The model under review builds one solid part; all positions refer to its coordinate system, in mm. Coordinates: 2 decimals unless noted, no trailing zeros. Loops run counter-clockwise (first coordinate to the right, second up) from the corner with the lowest first, then second, coordinate; pieces in that order, holes last. Notation, with made-up numbers: M -23.75,-17 L 35.25,-17 A28 ccw 35.25,8 Z; hole C 43,67 d2. An arc over 180 degrees is marked long. Return JSON: item names as keys, results as strings.
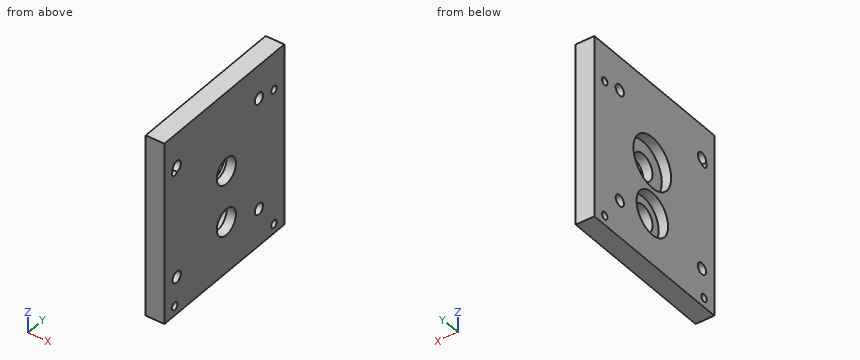
```python
from build123d import *

# Parameters (mm, degrees)
SKETCH1_W           = 20
SKETCH1_H           = 196
BOSS_EXTRUDE1_DEPTH = 175
SKETCH2_R           = 27.5
SKETCH2_R_2         = 23
CUT_EXTRUDE1_DEPTH  = 10
SKETCH3_R           = 14
CUT_EXTRUDE2_DEPTH  = 11
SKETCH4_R           = 4
CUT_EXTRUDE3_DEPTH  = 21
SKETCH5_R           = 6
CUT_EXTRUDE4_DEPTH  = 21


with BuildPart() as part:
    # Sketch1 → Boss-Extrude1 (new body)
    with BuildSketch(Plane(origin=(114, 0, 0), x_dir=(1, 0, 0), z_dir=(0, 1, 0))):
        with Locations((-114, 0)):
            Rectangle(SKETCH1_W, SKETCH1_H)
    extrude(amount=BOSS_EXTRUDE1_DEPTH)

    # Sketch2 → Cut-Extrude1 (cut)
    with BuildSketch(Plane.ZY.offset(10)):
        with Locations((12.5, 90.5)):
            Circle(SKETCH2_R)
        with Locations((-43, 90.5)):
            Circle(SKETCH2_R_2)
    extrude(amount=-CUT_EXTRUDE1_DEPTH, mode=Mode.SUBTRACT)

    # Sketch3 → Cut-Extrude2 (cut, through all)
    with BuildSketch(Plane.ZY):
        with Locations((12.5, 90.5)):
            Circle(SKETCH3_R)
        with Locations((-43, 90.5)):
            Circle(SKETCH3_R)
    extrude(amount=-CUT_EXTRUDE2_DEPTH, mode=Mode.SUBTRACT)

    # Sketch4 → Cut-Extrude3 (cut, through all)
    with BuildSketch(Plane.ZY.offset(10)):
        with Locations((58, 15)):
            Circle(SKETCH4_R)
        with Locations((-88, 15)):
            Circle(SKETCH4_R)
        with Locations((-88, 160)):
            Circle(SKETCH4_R)
        with Locations((58, 160)):
            Circle(SKETCH4_R)
    extrude(amount=-CUT_EXTRUDE3_DEPTH, mode=Mode.SUBTRACT)

    # Sketch5 → Cut-Extrude4 (cut, through all)
    with BuildSketch(Plane.ZY.offset(10)):
        with Locations((62, 138)):
            Circle(SKETCH5_R)
        with Locations((62, 18)):
            Circle(SKETCH5_R)
        with Locations((-58, 138)):
            Circle(SKETCH5_R)
        with Locations((-58, 18)):
            Circle(SKETCH5_R)
    extrude(amount=-CUT_EXTRUDE4_DEPTH, mode=Mode.SUBTRACT)


solid = part.part
```
1. Add section B-B on y = 138. Give the boundary of the cut face in (x, z).
Check values:
{"outline": "M -10,-98 L 10,-98 L 10,-64 L -10,-64 Z; M -10,-52 L 10,-52 L 10,56 L -10,56 Z; M -10,68 L 10,68 L 10,98 L -10,98 Z"}
2. Add section D-D on y = 107. Give the boundary of the cut face in (x, z), plus the area to 3 significant figures.
Check values:
{"outline": "M -10,-98 L 10,-98 L 10,98 L -10,98 L -10,34.5 L 0,34.5 L 0,-9.5 L -10,-9.5 L -10,-26.98 L 0,-26.98 L 0,-59.02 L -10,-59.02 Z", "area": "3,160 mm²"}
3. Insertion check: pin 1 Ø4 at (y, z) = (107.5, -42) entering from -X. The pin has a flat end and moves straight along its axis. Give the tip position at first contact, or say it passes through.
Check values:
{"pin 1": "x = 0"}
4. Add section A-A on z = 11.5. Give the boundary of the cut face in (x, y).
Check values:
{"outline": "M -10,0 L 10,0 L 10,76.54 L 0,76.54 L 0,63.02 L -10,63.02 Z; M -10,117.98 L 0,117.98 L 0,104.46 L 10,104.46 L 10,175 L -10,175 Z"}
5. To check wall thickness, follow line 1 (Y direction, x = -4.5, z = -88); line 2 (Z direction, x = 8, y = 143.5); line 3 (Z direction, x = -3.25, y = 79). State the ranges of each line that lie inside material, in increasing order.
Check values:
{"line 1": "0 to 11, 19 to 156, 164 to 175", "line 2": "-98 to -60.4, -55.6 to 59.6, 64.4 to 98", "line 3": "-98 to -62.92, -23.08 to -12.48, 37.48 to 98"}
6. Add section C-C on x = -4.5. State how many separate pieces and enclosed holes the cut face has, plus the area to 3 significant figures.
Check values:
{"separate pieces": "1", "enclosed holes": "9", "area": "29,600 mm²"}
